Design review of the part shown in the three views and the two pictorial views. Dimensions are in mm from the part's minimum x, y and z. Round coordinates to 2 decimals unless told otherwise and drop trailing zeros. Order: outer loops, then holes, each group sorted by start corner. A loop starts at its lowest first (then second) coordinate and runs counter-clockwise, first axis right, second up. Notation, with made-up numbers: (-17, 9.5) - (-2, 9.5) arc R24 cw to (-2, 27.5) - close; hole circle Ø3 at (-2.5, 27.5). An arc over 180 degrees is marked (long way). One line per question, with ' | ' between items. Start each with the question number.
Item 1: Add section A-A on y = 0.9. State how many separate pieces and enclosed holes the cut face has, and give its area (3 significant figures).
Item 2: Insertion check: pin 1 Ø1 at (y, z) = (2.5, 64) entering from -X; pin 2 Ø0.9 at (x, y) = (102.5, 2) entering from -Z; pin 3 Ø3.5 at (x, z) = (93, 25.5) entering from +Y; pin 4 Ø1 at (y, z) = (2.5, 71.5) entering from +X. Each pin has a flat end and moves straight along its axis. Give the tip position at first contact, or say it passes through.
Item 3: Add section C-C on x = 40. State the section outline as (y, z) points.
Item 4: Add section D-D on z = 25.5. State the section outline as (x, y) points, and give its area (3 significant figures).
Item 5: For L1, parallel to Z at x = 108, y = 1.8; L2, parallel to X at y = 1.9, z = 40; L3, parallel to X at y = 1.25, z = 54.5, list the stretches that pass through material, from the lowest coordinate up. Write a range as [from, to].
Item 6: Add section B-B on x = 108. State the section outline as (y, z) points.
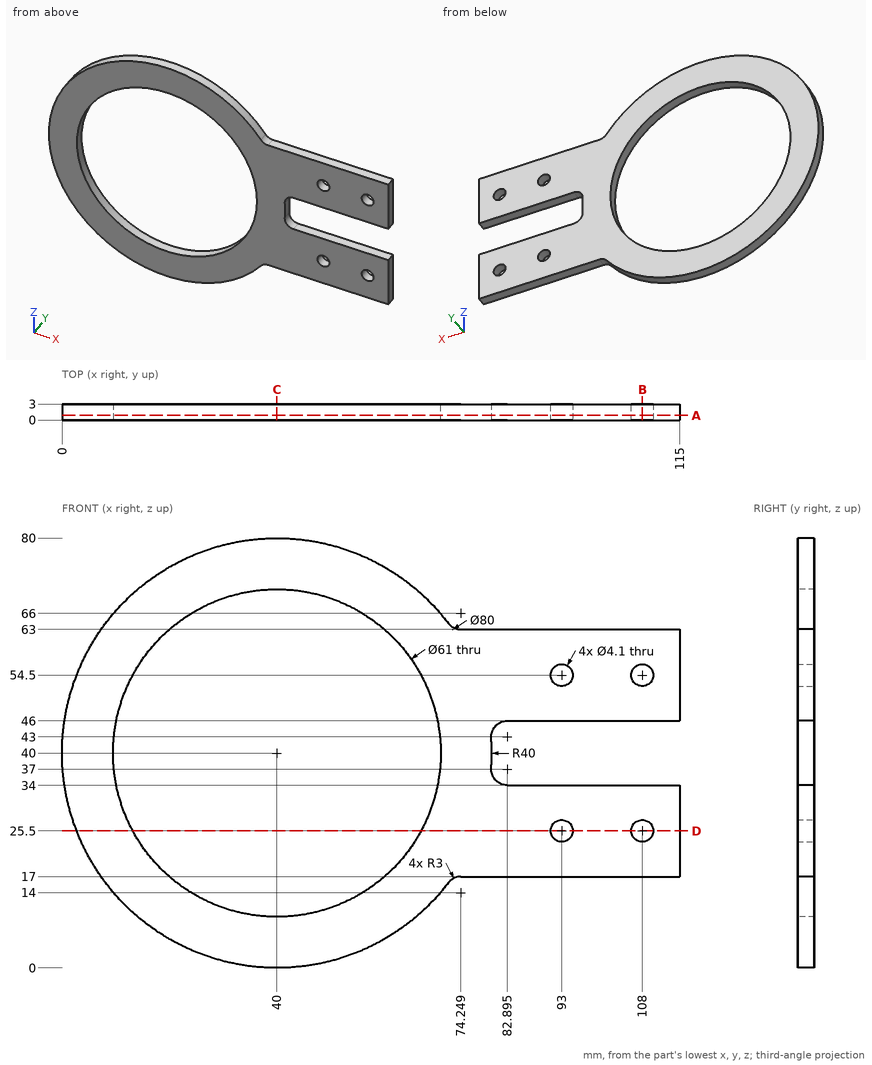
Determined:
1) separate pieces: 1 | enclosed holes: 5 | area: 3,350 mm2
2) pin 1: x = 7.63 | pin 2: z = 17 | pin 3: through | pin 4: x = 65.28
3) outline: (0, 0) - (3, 0) - (3, 9.5) - (0, 9.5) - close; (0, 70.5) - (3, 70.5) - (3, 80) - (0, 80) - close
4) outline: (2.72, 0) - (13.17, 0) - (13.17, 3) - (2.72, 3) - close; (66.83, 0) - (90.95, 0) - (90.95, 3) - (66.83, 3) - close; (95.05, 0) - (105.95, 0) - (105.95, 3) - (95.05, 3) - close; (110.05, 0) - (115, 0) - (115, 3) - (110.05, 3) - close | area: 151 mm2
5) L1: [17, 23.45], [27.55, 34], [46, 52.45], [56.55, 63] | L2: [0, 9.5], [70.5, 80] | L3: [2.72, 13.17], [66.83, 90.95], [95.05, 105.95], [110.05, 115]
6) outline: (0, 17) - (3, 17) - (3, 23.45) - (0, 23.45) - close; (0, 27.55) - (3, 27.55) - (3, 34) - (0, 34) - close; (0, 46) - (3, 46) - (3, 52.45) - (0, 52.45) - close; (0, 56.55) - (3, 56.55) - (3, 63) - (0, 63) - close
